Work out the finished part from the listing and answer in its coordinate system (mm). A direction names the side the tool comes from. Give positions to 0.01 mm unless a question says otherwise; leave off trailing zeros. Loops run counter-clockwise (first coordinate to the right, second up) from the corner with the lowest first, then second, coordinate; pieces in that order, holes last.
from build123d import *

# Parameters (mm, degrees)
PAD_DEPTH        = 3.2
THICKNESS_T      = -2
SKETCH026_R      = 1.25
POCKET010_DEPTH  = 3.201
CHAMFER001_ANGLE = 60
CHAMFER001_SIZE  = 0.8


with BuildPart() as part:
    # Sketch025 → Pad (new body)
    with BuildSketch(Plane(origin=(0, 0, 0), x_dir=(-1, 0, 0), z_dir=(0, 0, 1))):
        with BuildLine():
            Line((-23.4, -44.000002), (-23.4, -0.999999))
            ThreePointArc((-20, 2.4), (-22.404163, 1.404164), (-23.4, -0.999999))
            Line((-20, 2.4), (-0.999999, 2.4))
            ThreePointArc((2.4, -1), (1.404164, 1.404163), (-0.999999, 2.4))
            Line((2.4, -1), (2.4, -44.000002))
            ThreePointArc((-0.999999, -47.4), (1.404163, -46.404164), (2.4, -44.000002))
            Line((-0.999999, -47.4), (-20.000001, -47.4))
            ThreePointArc((-23.4, -44.000002), (-22.404163, -46.404164), (-20.000001, -47.4))
        make_face()
    extrude(amount=PAD_DEPTH)

    # Thickness
    thickness_openings = [part.faces().sort_by_distance(p)[0] for p in [
        (10.5, 22.5, 3.2),
    ]]
    offset(amount=THICKNESS_T, openings=thickness_openings)

    # Sketch026 (on Face9 of Thickness) → Pocket010 (cut, through all)
    with BuildSketch(Plane(origin=(0, 0, 0), x_dir=(1, 0, 0), z_dir=(0, 0, -1))):
        with Locations((3, -3)):
            Circle(SKETCH026_R)
        with Locations((18, -3)):
            Circle(SKETCH026_R)
        with Locations((18, -42)):
            Circle(SKETCH026_R)
        with Locations((3, -42)):
            Circle(SKETCH026_R)
    extrude(amount=-POCKET010_DEPTH, mode=Mode.SUBTRACT)

    # Chamfer001
    chamfer001_edges = [part.edges().sort_by_distance(p)[0] for p in [
        (1.75, 42, 0),
        (16.75, 42, 0),
        (1.75, 3, 0),
        (16.75, 3, 0),
    ]]
    chamfer001_side = part.faces().sort_by_distance((10.5, 22.5, 0))[0]
    chamfer(chamfer001_edges, length=CHAMFER001_SIZE, angle=CHAMFER001_ANGLE, reference=chamfer001_side)


with BuildPart() as part_1:
    # Body010 placement: moved
    add(part.part.moved(Location((0, 0, -3.6))))


solid = part_1.part
Item 1: Flat-ended cylindrical pins translate along their axes: pin 1 Ø8 at (x, y) = (7, 11) entering from +Z; pin 2 Ø10 at (x, y) = (19.5, 3.5) entering from -Z; pin 3 Ø3 at (x, y) = (18, 42) entering from -Z. Find the tip coordinate at first contact, or state that the pin passes through.
Item 2: Consider line 1 (Y direction, x = 18, z = -1.8); line 2 (X direction, y = 3, z = -1.75); line 3 (X direction, y = 28.5, z = -1.1). Determine where each line is inside the solid, lowest interval first.
Item 3: Find section D-D, the plane x = 14.75. Write down the section's boundary in (y, z).
Item 4: Find section C-C, the plane y = 14. Write down the section's boundary in (x, z), plus the area to 3 significant figures.
Item 5: Determine the mould class of faces 1 (the face through (-0.4, 22, -1)), 2 (the face through (22.43, 46.38, -2.02)), 3 (the face through (-2.4, 22, -2)) for opening direction X: released by +X, released by -X, zero draft, split by the parting line, or undercut.
Item 6: Find section A-A, the plane x = 18. Write down the section's boundary in (y, z).
Item 7: Find section B-B, the plane y = 42. Write down the section's boundary in (x, z).
Item 8: For faces 4 (the face through (21.4, 23, -1)), 5 (the face through (19.155, 42.479, -1.911)), determine the directions among +Z, -Z, +X, -X, +Y, -Y from which every point of the face is accessible in a straight line to the end or side of a thin tool.
Ans:
1. pin 1: stops at z = -1.6
1. pin 2: stops at z = -3.6
1. pin 3: stops at z = -2.65
2. line 1: y = -2.4 to 1.75, 4.25 to 40.75, 43.25 to 47.4
2. line 2: x = -2.4 to 1.75, 4.25 to 16.75, 19.25 to 23.4
2. line 3: x = -2.4 to -0.4, 21.4 to 23.4
3. outline: (-2.4, -3.6) - (47.4, -3.6) - (47.4, -0.4) - (45.4, -0.4) - (45.4, -1.6) - (-0.4, -1.6) - (-0.4, -0.4) - (-2.4, -0.4) - close
4. outline: (-2.4, -3.6) - (23.4, -3.6) - (23.4, -0.4) - (21.4, -0.4) - (21.4, -1.6) - (-0.4, -1.6) - (-0.4, -0.4) - (-2.4, -0.4) - close
4. area: 56.4 mm2
5. face 1: undercut
5. face 2: released by +X
5. face 3: released by -X
6. outline: (-2.4, -3.6) - (0.95, -3.6) - (1.75, -2.21) - (1.75, -1.6) - (-0.4, -1.6) - (-0.4, -0.4) - (-2.4, -0.4) - close; (4.25, -2.21) - (5.05, -3.6) - (39.95, -3.6) - (40.75, -2.21) - (40.75, -1.6) - (4.25, -1.6) - close; (43.25, -2.21) - (44.05, -3.6) - (47.4, -3.6) - (47.4, -0.4) - (45.4, -0.4) - (45.4, -1.6) - (43.25, -1.6) - close
7. outline: (-2.4, -3.6) - (0.95, -3.6) - (1.75, -2.21) - (1.75, -1.6) - (-0.4, -1.6) - (-0.4, -0.4) - (-2.4, -0.4) - close; (4.25, -2.21) - (5.05, -3.6) - (15.95, -3.6) - (16.75, -2.21) - (16.75, -1.6) - (4.25, -1.6) - close; (19.25, -2.21) - (20.05, -3.6) - (23.4, -3.6) - (23.4, -0.4) - (21.4, -0.4) - (21.4, -1.6) - (19.25, -1.6) - close
8. face 4: +Z
8. face 5: +Z, -Z
